Design review of the part built by this model. Coordinates are the model's own, in mm. A direction names the side the tool comes from. Coordinates: 2 decimals unless noted, no trailing zeros. Write each loop counter-clockwise with the first axis right and the second up, starting at its lowest first coordinate (ties: lowest second). Pieces come first, ordered by that corner, then holes. Notation, with made-up numbers: (-10, 46) - (-3, 46) arc R24 ccw to (-3, 73) - close; hole circle Ø10 at (72.25, 8.25). An arc over 180 degrees is marked (long way). Use a Markdown table: item, result.
from build123d import *

# Parameters (mm, degrees)
SKETCH1_R           = 19.675
BOSS_EXTRUDE1_DEPTH = 2.76
SKETCH2_W           = 2
SKETCH2_H           = 14
SKETCH2_W_2         = 14
SKETCH2_H_2         = 2
BOSS_EXTRUDE2_DEPTH = 155
SKETCH3_R           = 15.5
BOSS_EXTRUDE3_DEPTH = 19


with BuildPart() as part:
    # Sketch1 → Boss-Extrude1 (new body)
    with BuildSketch(Plane(origin=(0, 0, 0), x_dir=(1, 0, 0), z_dir=(0, 1, 0))):
        with Locations(Location((0, 0, 0), (0, 0, 270))):
            Circle(SKETCH1_R)
    extrude(amount=BOSS_EXTRUDE1_DEPTH)

    # Sketch2 → Boss-Extrude2 (add)
    with BuildSketch(Plane(origin=(0, 2.76, 0), x_dir=(1, 0, 0), z_dir=(0, 1, 0))):
        with Locations((0, 8)):
            Rectangle(SKETCH2_W, SKETCH2_H)
        with Locations((8, 0)):
            Rectangle(SKETCH2_W_2, SKETCH2_H_2)
        Rectangle(SKETCH2_W, SKETCH2_H_2)
        with Locations((0, -8)):
            Rectangle(SKETCH2_W, SKETCH2_H)
        with Locations((-8, 0)):
            Rectangle(SKETCH2_W_2, SKETCH2_H_2)
    extrude(amount=BOSS_EXTRUDE2_DEPTH)

    # Sketch3 → Boss-Extrude3 (add)
    with BuildSketch(Plane(origin=(0, 157.76, 0), x_dir=(1, 0, 0), z_dir=(0, 1, 0))):
        with Locations(Location((0, 0, 0), (0, 0, 270))):
            Circle(SKETCH3_R)
    extrude(amount=BOSS_EXTRUDE3_DEPTH)


solid = part.part
(1) Take a section at C-C on z = 17.5. Write out the cut boundary in (x, y), and give its area (3 significant figures).
Determined:
| item | result |
|---|---|
| outline | (-8.99, 0) - (8.99, 0) - (8.99, 2.76) - (-8.99, 2.76) - close |
| area | 49.6 mm2 |
(2) For pin 1 (7 mm diameter, centred on x = 5.5, y = 65.5, fed in from -Z); pin 2 (2 mm diameter, centred on x = 0, y = 75, fed in from +Z); pin 3 (2 mm diameter, centred on x = 7, y = 112, fed in from +Z), all flat-tipped, find the tip position at first contact; note any pin that passes through.
Determined:
| item | result |
|---|---|
| pin 1 | z = -1 |
| pin 2 | z = 15 |
| pin 3 | z = 1 |
(3) Take a section at B-B on z = -10. Write out the cut boundary in (x, y).
Determined:
| item | result |
|---|---|
| outline | (-16.94, 0) - (16.94, 0) - (16.94, 2.76) - (1, 2.76) - (1, 157.76) - (11.84, 157.76) - (11.84, 176.76) - (-11.84, 176.76) - (-11.84, 157.76) - (-1, 157.76) - (-1, 2.76) - (-16.94, 2.76) - close |
(4) Draft analysis for pull direction Y (two halves, no side actions). For faces 5 (the cylindrical face through (15.368, 167.127, -2.018)), 6 (the flat face through (8, 79, -1)), 7 (the flat face through (0, 176.76, 0)), state which applies: +Y half, -Y half, draft (parallel to the pull), parting line (faces both ways), or undercut.
Determined:
| item | result |
|---|---|
| face 5 | draft |
| face 6 | undercut |
| face 7 | +Y half |
(5) For L1, parallel to Y at x = 6, z = 2.5; L2, parallel to X at y = 10, z = -8.5; L3, parallel to Y at x = 16, z = 3.5, list the stretches that pass through material, from the lowest coordinate up. Write a range as from..to.
Determined:
| item | result |
|---|---|
| L1 | 0..2.76, 157.76..176.76 |
| L2 | -1..1 |
| L3 | 0..2.76 |
(6) Take a section at A-A on y = 83. Write out the cut boundary in (x, z), and give its area (3 significant figures).
Determined:
| item | result |
|---|---|
| outline | (-15, -1) - (-1, -1) - (-1, -15) - (1, -15) - (1, -1) - (15, -1) - (15, 1) - (1, 1) - (1, 15) - (-1, 15) - (-1, 1) - (-15, 1) - close |
| area | 116 mm2 |
(7) Machinability: for faces 1 (the flat face through (1, 79, 8)), 2 (the flat face through (-3, 157.76, 3)), 3 (the flat face through (-1, 79, 8)), 4 (the flat face through (-8, 79, -1)), which of the approach directions +Z, -Z, +X, -X, +Y, -Y give a long, thin tool a straight path to every point of the face, cutting with its end or side? Answer none if there is none.
Determined:
| item | result |
|---|---|
| face 1 | +Z, +X |
| face 2 | none |
| face 3 | +Z, -X |
| face 4 | -Z, -X |
